Source: three-view drawing plus pictorial views. Frame: mm from the lowest corner of the part. Give positions to 0.01 mm unless a question says otherwise; leave off trailing zeros. Order: outer loops, then holes, each group sorted by start corner. A loop starts at its lowest first (then second) coordinate and runs counter-clockwise, first axis right, second up. Notation, with made-up numbers: (15, 87.25) - (66, 87.25) arc R12 ccw to (66, 108.25) - close; hole circle Ø1 at (17.25, 86). An arc over 180 degrees is marked (long way). Use one line per item in the form item = value.
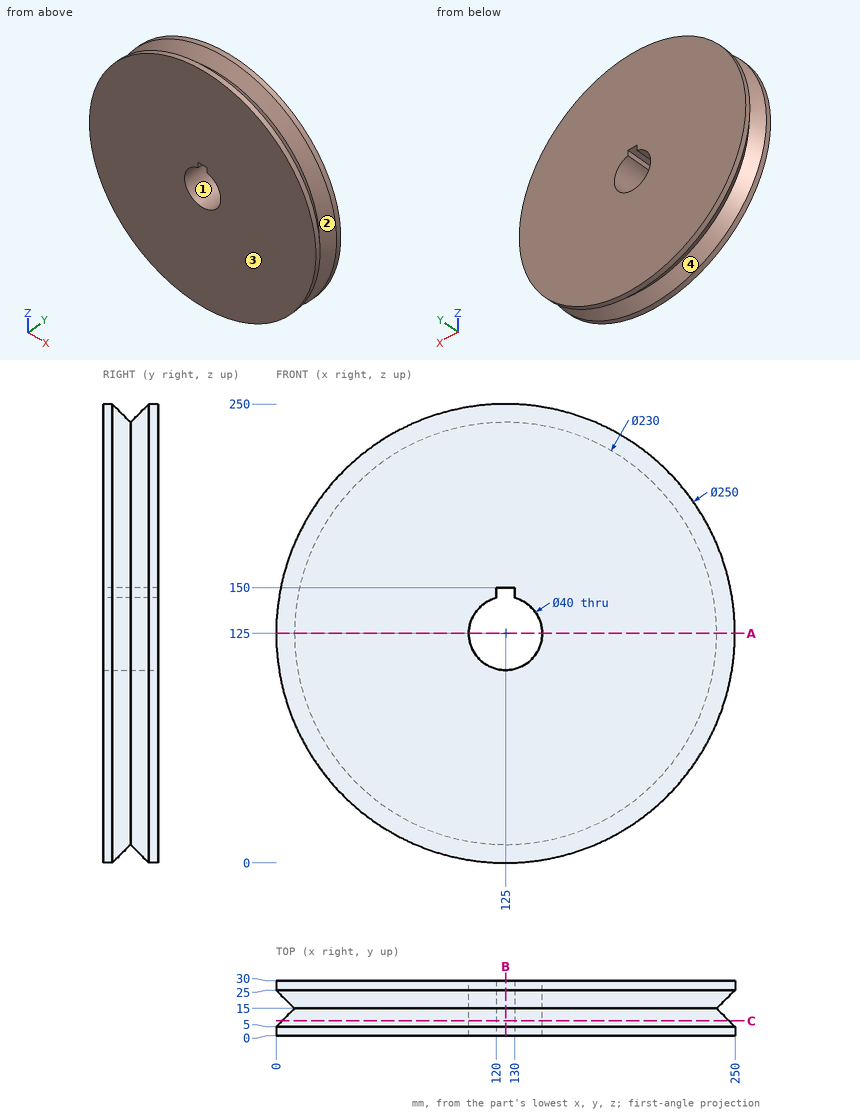
(1) Ray query, line 1 along X through (y, z) = (8.25, 121.5); line 2 along X through (y, z) = (24, 142.5); line 3 along Z through (x, y) = (135.5, 18.5). Return the intervals inside material, ascending.
Computed values:
line_1 = 3.3 to 105.31, 144.69 to 246.7
line_2 = 2.24 to 115.32, 134.68 to 247.76
line_3 = 6.97 to 107.98, 142.02 to 243.03
(2) Cut plane A-A on z = 125. Output: boundary loops of the cut face in (x, y).
Computed values:
outline = (0, 0) - (105, 0) - (105, 30) - (0, 30) - (0, 25) - (10, 15) - (0, 5) - close; (145, 0) - (250, 0) - (250, 5) - (240, 15) - (250, 25) - (250, 30) - (145, 30) - close
(3) Pull-direction query (Y, two-part tool) for the marked faces 1, 2, 3 and 4; classes: released by +Y, released by -Y, zero draft, split by the parting line, or undercut.
Computed values:
face_1 = zero draft
face_2 = undercut
face_3 = released by -Y
face_4 = undercut
(4) Cut plane B-B on x = 125. Output: boundary loops of the cut face in (y, z), plus the area to 3 significant figures.
Computed values:
outline = (0, 0) - (5, 0) - (15, 10) - (25, 0) - (30, 0) - (30, 105) - (0, 105) - close; (0, 150) - (30, 150) - (30, 250) - (25, 250) - (15, 240) - (5, 250) - (0, 250) - close
area = 5,950 mm²
(5) Contact query for flat-ended pins moving along their axis: pin 1 Ø12 at (x, z) = (83, 50.5) entering from -Y; pin 2 Ø4.5 at (y, z) = (15, 146) entering from +X; pin 3 Ø3 at (y, z) = (26.5, 214.5) entering from +X (3 decimals); pin 4 Ø4 at (x, y) = (59.5, 19.5) entering from -Z. Output: stop coordinate, or through.
Computed values:
pin_1 = 0
pin_2 = 240.39
pin_3 = 213.775
pin_4 = 22.35
(6) Cut plane C-C on y = 8.25. Output: boundary loops of the cut face in (x, z), plus the area to 3 significant figures.
Computed values:
outline = circle Ø243.5 at (125, 125); hole (120, 144.36) arc R20 ccw (long way) to (130, 144.36) - (130, 150) - (120, 150) - close
area = 45,300 mm²
